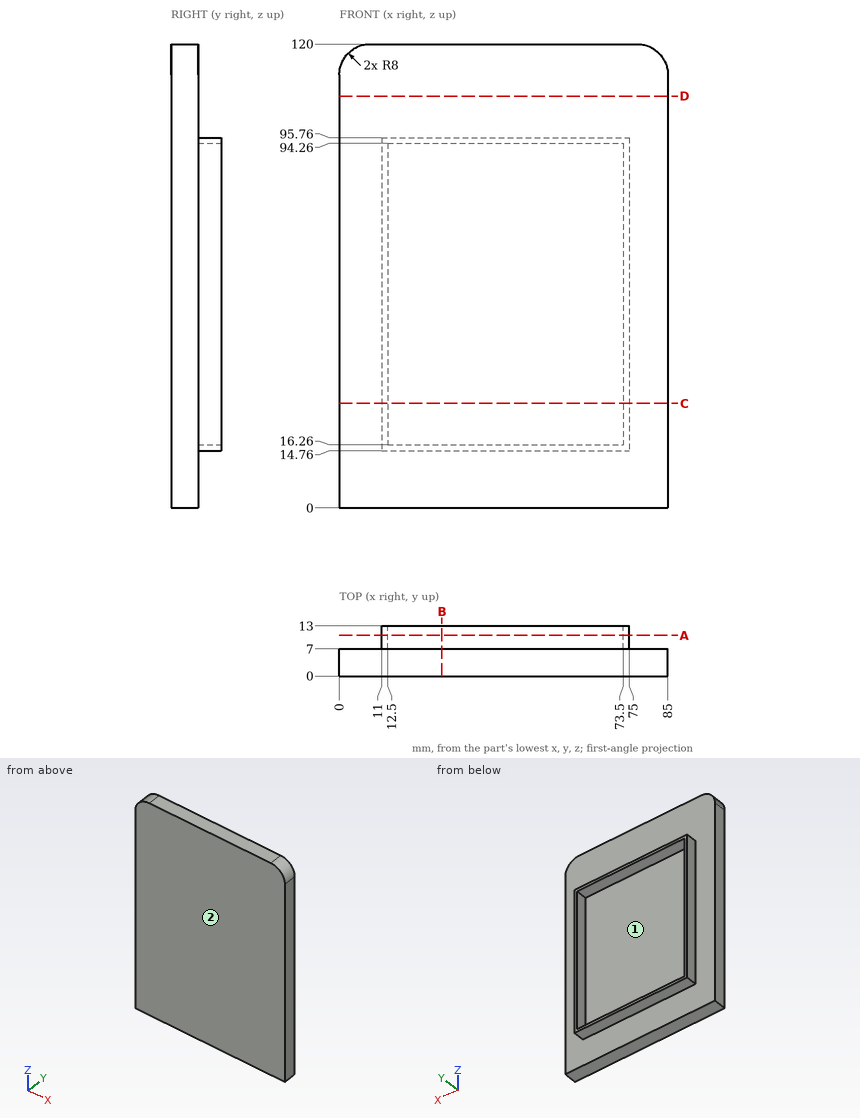
Answer from the drawing. Dimensions are ordinates in mm from the lowest x, y and z of the part. Round coordinates to 2 decimals unless told otherwise and drop trailing zeros. Order: outer loops, then holes, each group sorted by start corner. A loop starts at its lowest first (then second) coordinate and runs counter-clockwise, first axis right, second up.
1) The mould has two halves that part along X. Classify the marked faces 1 and 2: released by +X, released by -X, zero draft, split by the parting line, or undercut.
2) The part is cut by section C-C on z = 27. Write down the section's boundary in (x, y).
3) The part is cut by section D-D on z = 106.5. Write down the section's boundary in (x, y), plus the area to 3 significant figures.
4) The part is cut by section A-A on y = 10.5. Write down the section's boundary in (x, z).
5) The part is cut by section B-B on x = 26.5. Write down the section's boundary in (y, z), plus the area to 3 significant figures.
6) Straight lines are drawn through the part: L1, parallel to Z at x = 38.5, y = 8; L2, parallel to Y at x = 27, z = 11; L3, parallel to X at y = 10.25, z = 83. For each, find the intervals that lie inside material, in ascending order.
7) Flat-ended cylindrical pins translate along their axes: pin 1 (5 mm diameter, centred on y = 11.5, z = 62.5, fed in from -X); pin 2 (6.5 mm diameter, centred on x = 37, y = 11, fed in from +Z); pin 3 (1.8 mm diameter, centred on x = 58, y = 10, fed in from -Z). Find the tip coordinate at first contact, or state that the pin passes through.
Resolved:
1. face 1: undercut
1. face 2: zero draft
2. outline: (0, 0) - (85, 0) - (85, 7) - (75, 7) - (75, 13) - (73.5, 13) - (73.5, 7) - (12.5, 7) - (12.5, 13) - (11, 13) - (11, 7) - (0, 7) - close
3. outline: (0, 0) - (85, 0) - (85, 7) - (0, 7) - close
3. area: 595 mm2
4. outline: (11, 14.76) - (75, 14.76) - (75, 95.76) - (11, 95.76) - close; hole (12.5, 16.26) - (73.5, 16.26) - (73.5, 94.26) - (12.5, 94.26) - close
5. outline: (0, 0) - (7, 0) - (7, 14.76) - (13, 14.76) - (13, 16.26) - (7, 16.26) - (7, 94.26) - (13, 94.26) - (13, 95.76) - (7, 95.76) - (7, 120) - (0, 120) - close
5. area: 858 mm2
6. L1: z = 14.76 to 16.26, 94.26 to 95.76
6. L2: y = 0 to 7
6. L3: x = 11 to 12.5, 73.5 to 75
7. pin 1: stops at x = 11
7. pin 2: stops at z = 95.76
7. pin 3: stops at z = 14.76
